from build123d import *

# Parameters (mm, degrees)
SKETCH18_W           = 228.04
SKETCH18_H           = 171.92
BOSS_EXTRUDE6_DEPTH  = 26.5
SKETCH20_W           = 218.04
SKETCH20_H           = 171.92
CUT_EXTRUDE6_DEPTH   = 21.5
SKETCH22_W           = 228.04
SKETCH22_H           = 18.7
BOSS_EXTRUDE7_DEPTH  = 26.5
SKETCH23_W           = 228.04
SKETCH23_H           = 18.7
BOSS_EXTRUDE8_DEPTH  = 26.5
SKETCH24_W           = 175
SKETCH24_H           = 18.7
CUT_EXTRUDE7_DEPTH   = 3.35
SKETCH25_W           = 175
SKETCH25_H           = 18.7
CUT_EXTRUDE8_DEPTH   = 3.35
SKETCH27_W           = 175
SKETCH27_H           = 12.7
CUT_EXTRUDE9_DEPTH   = 3
SKETCH28_W           = 175
SKETCH28_H           = 12.7
CUT_EXTRUDE10_DEPTH  = 3
SKETCH31_R           = 1.65
SKETCH31_R_2         = 1.651
CUT_EXTRUDE15_DEPTH  = 1.825
CUT_EXTRUDE17_DEPTH  = 3.175
SKETCH38_R           = 2.75
BOSS_EXTRUDE12_DEPTH = 8
SKETCH39_R           = 2.2
CUT_EXTRUDE18_DEPTH  = 26.5
SKETCH40_R           = 4.4
CUT_EXTRUDE19_DEPTH  = 20.9
FILLET1_R            = 3.81
CUT_EXTRUDE20_DEPTH  = 3.6
SKETCH47_R           = 3.3782
BOSS_EXTRUDE14_DEPTH = 10.16


with BuildPart() as part:
    # Sketch18 → Boss-Extrude6 (new body)
    with BuildSketch(Plane(origin=(0, 0, 0), x_dir=(1, 0, 0), z_dir=(0, 1, 0))):
        Rectangle(SKETCH18_W, SKETCH18_H)
    extrude(amount=BOSS_EXTRUDE6_DEPTH)

    # Sketch20 → Cut-Extrude6 (cut)
    with BuildSketch(Plane(origin=(0, 26.5, 0), x_dir=(1, 0, 0), z_dir=(0, 1, 0))):
        Rectangle(SKETCH20_W, SKETCH20_H)
    extrude(amount=-CUT_EXTRUDE6_DEPTH, mode=Mode.SUBTRACT)

    # Sketch22 → Boss-Extrude7 (add)
    with BuildSketch(Plane(origin=(0, 0, 0), x_dir=(1, 0, 0), z_dir=(0, 1, 0))):
        with Locations((0, -95.31)):
            Rectangle(SKETCH22_W, SKETCH22_H)
    extrude(amount=BOSS_EXTRUDE7_DEPTH)

    # Sketch23 → Boss-Extrude8 (add)
    with BuildSketch(Plane(origin=(0, 0, 0), x_dir=(1, 0, 0), z_dir=(0, 1, 0))):
        with Locations((0, 95.31)):
            Rectangle(SKETCH23_W, SKETCH23_H)
    extrude(amount=BOSS_EXTRUDE8_DEPTH)

    # Sketch24 → Cut-Extrude7 (cut)
    with BuildSketch(Plane(origin=(0, 26.5, 0), x_dir=(1, 0, 0), z_dir=(0, 1, 0))):
        with Locations((0, 95.31)):
            Rectangle(SKETCH24_W, SKETCH24_H)
    extrude(amount=-CUT_EXTRUDE7_DEPTH, mode=Mode.SUBTRACT)

    # Sketch25 → Cut-Extrude8 (cut)
    with BuildSketch(Plane(origin=(0, 26.5, 0), x_dir=(1, 0, 0), z_dir=(0, 1, 0))):
        with Locations((0, -95.31)):
            Rectangle(SKETCH25_W, SKETCH25_H)
    extrude(amount=-CUT_EXTRUDE8_DEPTH, mode=Mode.SUBTRACT)

    # Sketch27 → Cut-Extrude9 (cut)
    with BuildSketch(Plane(origin=(0, 23.15, 0), x_dir=(1, 0, 0), z_dir=(0, 1, 0))):
        with Locations((0, -95.31)):
            Rectangle(SKETCH27_W, SKETCH27_H)
    extrude(amount=-CUT_EXTRUDE9_DEPTH, mode=Mode.SUBTRACT)

    # Sketch28 → Cut-Extrude10 (cut)
    with BuildSketch(Plane(origin=(0, 23.15, 0), x_dir=(1, 0, 0), z_dir=(0, 1, 0))):
        with Locations((0, 95.31)):
            Rectangle(SKETCH28_W, SKETCH28_H)
    extrude(amount=-CUT_EXTRUDE10_DEPTH, mode=Mode.SUBTRACT)

    # Sketch31 → Cut-Extrude15 (cut)
    with BuildSketch(Plane(origin=(0, 5, 0), x_dir=(1, 0, 0), z_dir=(0, 1, 0))):
        with Locations(Location((-82.448, 57.15, 0), (0, 0, 270))):
            Circle(SKETCH31_R)
        with Locations(Location((101.448, 57.15, 0), (0, 0, 270))):
            Circle(SKETCH31_R_2)
        with Locations(Location((101.448, -57.15, 0), (0, 0, 270))):
            Circle(SKETCH31_R_2)
        with Locations(Location((-82.448, -57.15, 0), (0, 0, 270))):
            Circle(SKETCH31_R)
    extrude(amount=-CUT_EXTRUDE15_DEPTH, mode=Mode.SUBTRACT)

    # Sketch33 → Cut-Extrude17 (cut)
    with BuildSketch(Plane.XZ):
        Polygon((-79.316971755, -58.9577), (-79.316971755, -55.3423), (-82.448, -53.5346), (-85.579028245, -55.3423), (-85.579028245, -58.9577), (-82.448, -60.7654), align=None)
        Polygon((104.579028245, -58.9577), (104.579028245, -55.3423), (101.448, -53.5346), (98.316971755, -55.3423), (98.316971755, -58.9577), (101.448, -60.7654), align=None)
        Polygon((-79.316971755, 58.9577), (-82.448, 60.7654), (-85.579028245, 58.9577), (-85.579028245, 55.3423), (-82.448, 53.5346), (-79.316971755, 55.3423), align=None)
        Polygon((98.316971755, 58.9577), (98.316971755, 55.3423), (101.448, 53.5346), (104.579028245, 55.3423), (104.579028245, 58.9577), (101.448, 60.7654), align=None)
    extrude(amount=-CUT_EXTRUDE17_DEPTH, mode=Mode.SUBTRACT)

    # Sketch38 → Boss-Extrude12 (add, symmetric)
    with BuildSketch(Plane.XY.offset(-52.33)):
        with BuildLine():
            Line((-114.02, 0), (-134.455863104, 20.352550116))
            ThreePointArc((-134.455863104, 20.352550116), (-135.406416884, 31.696896104), (-124.062070896, 32.647449884))
            Line((-124.062070896, 32.647449884), (-114.02, 26.5))
            Line((-114.02, 26.5), (-114.02, 0))
        make_face()
        with Locations((-129.258967, 26.5)):
            Circle(SKETCH38_R, mode=Mode.SUBTRACT)
    boss_extrude12 = extrude(amount=BOSS_EXTRUDE12_DEPTH, both=True)

    # Mirror2: Boss-Extrude12 across plane
    add(boss_extrude12.mirror(Plane.XY))

    # Sketch39 → Cut-Extrude18 (cut)
    with BuildSketch(Plane(origin=(0, 26.5, 0), x_dir=(1, 0, 0), z_dir=(0, 1, 0))):
        with Locations(Location((100.76, 95.31, 0), (0, 0, 270))):
            Circle(SKETCH39_R)
    cut_extrude18 = extrude(amount=-CUT_EXTRUDE18_DEPTH, mode=Mode.SUBTRACT)

    # Sketch40 → Cut-Extrude19 (cut)
    with BuildSketch(Plane.XZ):
        with Locations(Location((100.76, -95.31, 0), (0, 0, 270))):
            Circle(SKETCH40_R)
    cut_extrude19 = extrude(amount=-CUT_EXTRUDE19_DEPTH, mode=Mode.SUBTRACT)

    # Mirror3: Cut-Extrude18 across plane
    add(cut_extrude18.mirror(Plane.XY), mode=Mode.SUBTRACT)

    # Mirror4: Cut-Extrude19 across plane
    add(cut_extrude19.mirror(Plane.XY), mode=Mode.SUBTRACT)

    # Fillet1
    fillet1_edges = [part.edges().sort_by_distance(p)[0] for p in [
        (-114.02, 13.25, 104.66),
        (114.02, 13.25, 104.66),
        (114.02, 13.25, -104.66),
        (-114.02, 13.25, -104.66),
    ]]
    fillet(fillet1_edges, radius=FILLET1_R)

    # Sketch41 → Cut-Extrude20 (cut)
    with BuildSketch(Plane(origin=(0, 26.5, 0), x_dir=(1, 0, 0), z_dir=(0, 1, 0))):
        Polygon((98.681539031, -91.71), (96.603078062, -95.31), (98.681539031, -98.91), (102.838460969, -98.91), (104.916921938, -95.31), (102.838460969, -91.71), align=None)
    cut_extrude20 = extrude(amount=-CUT_EXTRUDE20_DEPTH, mode=Mode.SUBTRACT)

    # Mirror5: Cut-Extrude20 across plane
    add(cut_extrude20.mirror(Plane.XY), mode=Mode.SUBTRACT)

    # Sketch47 → Boss-Extrude14 (add)
    # profile 1 of 2: a face of its own
    with BuildSketch(Plane.XZ):
        with BuildLine():
            ThreePointArc((-48.903154853, -113.757225166), (-47.210651626, -109.12978233), (-45.13728714, -104.66))
            Line((-45.13728714, -104.66), (-57.122870876, -104.66))
            Line((-57.122870876, -104.66), (-68.88271286, -104.66))
            ThreePointArc((-68.88271286, -104.66), (-66.809348374, -109.12978233), (-65.116845147, -113.757225166))
            ThreePointArc((-65.116845147, -113.757225166), (-57.01, -120.350559583), (-48.903154853, -113.757225166))
        make_face()
        with Locations(Location((-57.01, -112.07, 0), (0, 0, 270))):
            Circle(SKETCH47_R, mode=Mode.SUBTRACT)
    # profile 2 of 2: a face of its own
    with BuildSketch(Plane.XZ):
        with BuildLine():
            ThreePointArc((45.13728714, -104.66), (47.210651626, -109.12978233), (48.903154853, -113.757225166))
            ThreePointArc((48.903154853, -113.757225166), (57.01, -120.350559583), (65.116845147, -113.757225166))
            ThreePointArc((65.116845147, -113.757225166), (66.809348374, -109.12978233), (68.88271286, -104.66))
            Line((68.88271286, -104.66), (57.122870876, -104.66))
            Line((57.122870876, -104.66), (45.13728714, -104.66))
        make_face()
        with Locations(Location((57.01, -112.07, 0), (0, 0, 270))):
            Circle(SKETCH47_R, mode=Mode.SUBTRACT)
    boss_extrude14 = extrude(amount=-BOSS_EXTRUDE14_DEPTH)

    # Mirror6: Boss-Extrude14 across plane
    add(boss_extrude14.mirror(Plane.XY))


solid = part.part
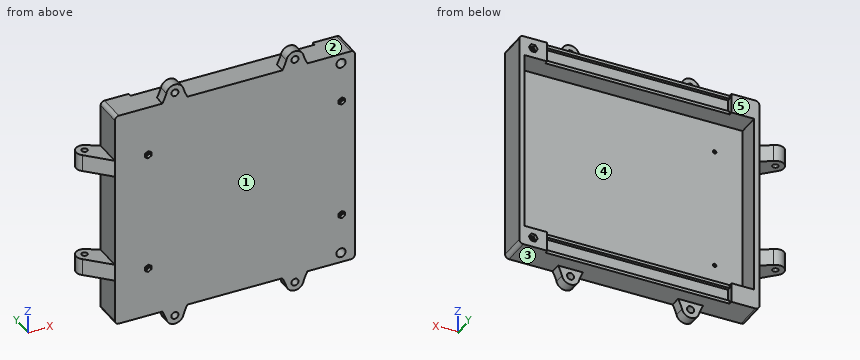
Verification items for the finished model (mm, model axes). Face numbers are marked on the shaded views. A direction names the side the tool comes from. Coordinates: 2 decimals unless noted, no trailing zeros. Write each loop counter-clockwise with the first axis right and the second up, starting at its lowest first coordinate (ties: lowest second). Pieces come first, ordered by that corner, then holes. Notation, with made-up numbers: M 35.5,61.25 L 73.5,61.25 A27 ccw 73.5,84.25 Z; hole C 29.5,5.25 d5. An arc over 180 degrees is marked long. Use CSV: the item, a comma, the result in double quotes.
Q1. Thickness scan on line 1 along Z through (x, y) = (-49, 16); line 2 along Z through (x, y) = (47, 7); line 3 along X through (y, z) = (15, 27). Record the ranges inside material, lowest first. Write a range as [from, to].
Computed values:
line 1,"[-104.66, -85.96], [85.96, 104.66]"
line 2,"[-108.63, -85.96], [85.96, 108.63]"
line 3,"[-114.02, -109.02], [109.02, 114.02]"
Q2. Section check C-C, the plane z = -20. Enter the section's corners in (x, y), and give its area (3 significant figures).
Computed values:
outline,"M -114.02,0 L 114.02,0 L 114.02,26.5 L 109.02,26.5 L 109.02,5 L -109.02,5 L -109.02,26.5 L -114.02,26.5 Z"
area,"1,360 mm²"
Q3. Mould release check, pull along X, two halves, no side actions. Record for the marked faces 1 and 2: pulls with the +X half, pulls with the -X half, needs draft (parallel to the pull), parting line crosses it, or undercut.
Computed values:
face 1,"needs draft"
face 2,"undercut"
Q4. Go/stop test with flat-tipped pins: P1, Ø1, axis at x = 48, y = 12, coming from the +Z side; P2, Ø0.9, axis at x = 33.5, y = 21.5, coming from the -Z side; P3, Ø10, axis at x = -91.5, z = -39, coming from the +Y side. Record where each tip stops, or that it passes through.
Computed values:
P1,"z = 104.66"
P2,"z = -104.66"
P3,"y = 5"
Q5. Section check D-D, the plane x = -5.5. Enter the section's corners in (y, z).
Computed values:
outline,"M 0,-104.66 L 23.15,-104.66 L 23.15,-101.66 L 20.15,-101.66 L 20.15,-88.96 L 23.15,-88.96 L 23.15,-85.96 L 5,-85.96 L 5,85.96 L 23.15,85.96 L 23.15,88.96 L 20.15,88.96 L 20.15,101.66 L 23.15,101.66 L 23.15,104.66 L 0,104.66 Z"
Q6. Section check B-B, the plane y = 17. Enter the section's corners in (x, z).
Computed values:
outline,"M -131.09,-60.33 L -114.02,-60.33 L -114.02,-100.85 A3.81 ccw -110.21,-104.66 L 110.21,-104.66 A3.81 ccw 114.02,-100.85 L 114.02,100.85 A3.81 ccw 110.21,104.66 L -110.21,104.66 A3.81 ccw -114.02,100.85 L -114.02,60.33 L -131.09,60.33 L -131.09,44.33 L -114.02,44.33 L -114.02,-44.33 L -131.09,-44.33 Z; hole M -109.02,-85.96 L 109.02,-85.96 L 109.02,85.96 L -109.02,85.96 Z; hole C 100.76,-95.31 d8.8; hole C 100.76,95.31 d8.8"
Q7. Section check A-A, the plane x = -57.01. Enter the section's corners in (y, z).
Computed values:
outline,"M 0,-120.35 L 10.16,-120.35 L 10.16,-115.45 L 0,-115.45 Z; M 0,-108.69 L 10.16,-108.69 L 10.16,-104.66 L 23.15,-104.66 L 23.15,-101.66 L 20.15,-101.66 L 20.15,-88.96 L 23.15,-88.96 L 23.15,-85.96 L 5,-85.96 L 5,85.96 L 23.15,85.96 L 23.15,88.96 L 20.15,88.96 L 20.15,101.66 L 23.15,101.66 L 23.15,104.66 L 10.16,104.66 L 10.16,108.69 L 0,108.69 Z; M 0,115.45 L 10.16,115.45 L 10.16,120.35 L 0,120.35 Z"
Q8. Set-up check for the marked faces 3, 4 and 5: record each of +Z, -Z, +X, -X, +Y, -Y from which the full face is reachable in a straight line by a thin tool's end or side.
Computed values:
face 3,"-Z, +Y"
face 4,"+Y"
face 5,"+Z, -Z, +X, +Y"
